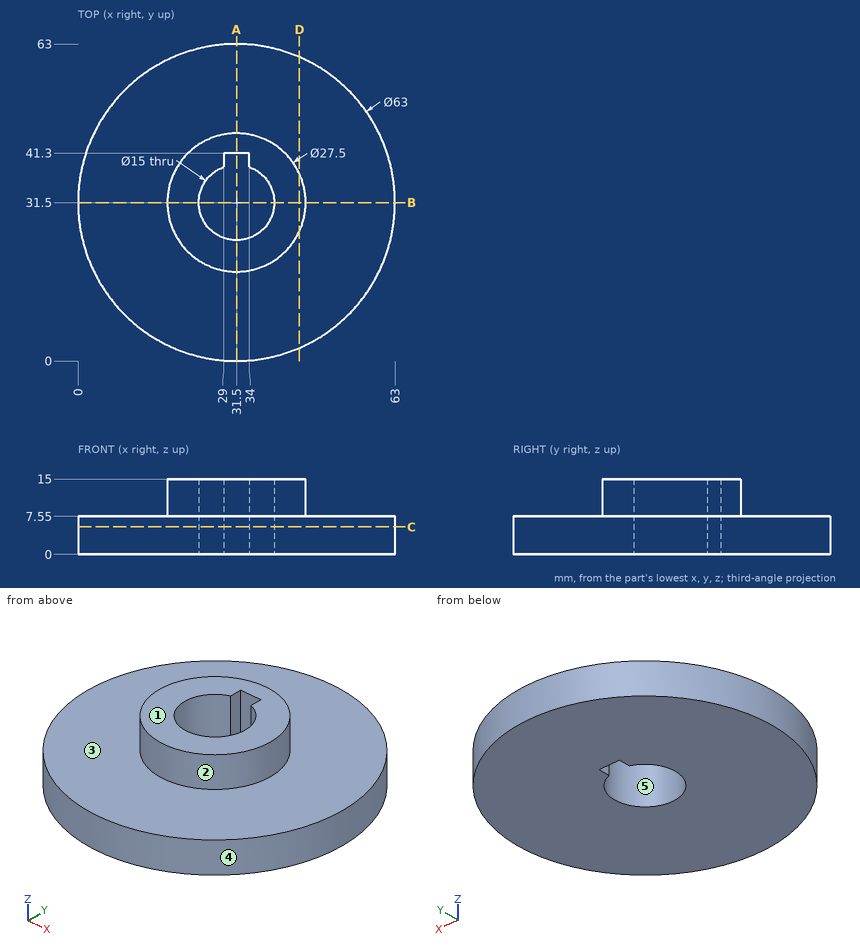
Design review of the part shown in the three views and the two pictorial views. Dimensions are in mm from the part's minimum x, y and z. A direction names the side the tool comes from. Round coordinates to 2 decimals unless told otherwise and drop trailing zeros. Loops run counter-clockwise (first coordinate to the right, second up) from the corner with the lowest first, then second, coordinate; pieces in that order, holes last. Notation, with made-up numbers: (37.25, 47.5) - (78.25, 47.5) arc R15 cw to (78.25, 54.5) - close; hole circle Ø9 at (-9, 67.5). An arc over 180 degrees is marked (long way). One line per item, written item: value. Start each with the question number.
Item 1: For L1, parallel to Y at x = 31.5, z = 5; L2, parallel to Z at x = 17, y = 44.5; L3, parallel to Y at x = 38, z = 12.75, list the stretches that pass through material, from the lowest coordinate up.
Item 2: Take a section at B-B (y = 31.5). Give the boundary of the cut face in (x, z).
Item 3: Take a section at C-C (z = 5.5). Give the boundary of the cut face in (x, y).
Item 4: Clearance check with flat-ended pins moving along their axes: pin 1 Ø3 at (y, z) = (40, 10) entering from -X; pin 2 Ø6 at (x, y) = (30.5, 54) entering from +Z; pin 3 Ø4 at (x, z) = (31.5, 11) entering from -Y; pin 4 Ø12 at (x, y) = (31.5, 31.5) entering from -Z. State where each tip first meets the part, or that it passes through.
Item 5: For the marked faces 1 and 2, list the 3-axis set-ups (+Z, -Z, +X, -X, +Y, -Y) from which the entire face can be reached by the end or side of a thin tool; tool diameter is ignored.
Item 6: Take a section at D-D (x = 44). Give the boundary of the cut face in (y, z).
Item 7: Take a section at A-A (x = 31.5). Give the boundary of the cut face in (y, z), plus the area to 3 significant figures.
Item 8: The part is to be moulded in two halves that separate along X. For the marked faces 3, 4 and 5, say which applies: +X half, -X half, draft (parallel to the pull), parting line (faces both ways), or undercut.
Answer below:
1. L1: y = 0 to 24, 41.3 to 63
1. L2: z = 0 to 7.55
1. L3: y = 19.38 to 27.76, 35.24 to 43.62
2. outline: (0, 0) - (24, 0) - (24, 15) - (17.75, 15) - (17.75, 7.55) - (0, 7.55) - close; (39, 0) - (63, 0) - (63, 7.55) - (45.25, 7.55) - (45.25, 15) - (39, 15) - close
3. outline: circle Ø63 at (31.5, 31.5); hole (29, 38.57) arc R7.5 ccw (long way) to (34, 38.57) - (34, 41.3) - (29, 41.3) - close
4. pin 1: stops at x = 19.67
4. pin 2: stops at z = 7.55
4. pin 3: stops at y = 17.75
4. pin 4: passes through
5. face 1: +Z, +X, -X, +Y, -Y
5. face 2: +Z
6. outline: (2.59, 0) - (60.41, 0) - (60.41, 7.55) - (37.23, 7.55) - (37.23, 15) - (25.77, 15) - (25.77, 7.55) - (2.59, 7.55) - close
7. outline: (0, 0) - (24, 0) - (24, 15) - (17.75, 15) - (17.75, 7.55) - (0, 7.55) - close; (41.3, 0) - (63, 0) - (63, 7.55) - (45.25, 7.55) - (45.25, 15) - (41.3, 15) - close
7. area: 421 mm2
8. face 3: draft
8. face 4: parting line
8. face 5: undercut
